from build123d import *

# Parameters (mm, degrees)
SKETCH1_R           = 2
SKETCH1_R_2         = 5
SKETCH1_R_3         = 1.55
SKETCH1_W           = 20
SKETCH1_H           = 7
BOSS_EXTRUDE1_DEPTH = 6


with BuildPart() as part:
    # Sketch1 → Boss-Extrude1 (new body)
    with BuildSketch(Plane.XY):
        with BuildLine():
            Line((95, -44.105037838), (35, -44.105037838))
            ThreePointArc((35, -44.105037838), (27.928932188, -41.17610565), (25, -34.105037838))
            Line((25, -34.105037838), (25, 41.105037842))
            ThreePointArc((25, 41.105037842), (25.732233047, 42.872804795), (27.5, 43.605037842))
            Line((27.5, 43.605037842), (45.75, 43.605037842))
            ThreePointArc((45.75, 43.605037842), (47.517766953, 44.337270889), (48.25, 46.105037842))
            Line((48.25, 46.105037842), (48.25, 61.605037842))
            ThreePointArc((48.25, 61.605037842), (47.517766953, 63.372804795), (45.75, 64.105037842))
            Line((45.75, 64.105037842), (-45.75, 64.105037842))
            ThreePointArc((-45.75, 64.105037842), (-47.517766953, 63.372804795), (-48.25, 61.605037842))
            Line((-48.25, 61.605037842), (-48.25, 46.105037842))
            ThreePointArc((-48.25, 46.105037842), (-47.517766953, 44.337270889), (-45.75, 43.605037842))
            Line((-45.75, 43.605037842), (-27.5, 43.605037842))
            ThreePointArc((-27.5, 43.605037842), (-25.732233047, 42.872804795), (-25, 41.105037842))
            Line((-25, 41.105037842), (-25, -34.105037838))
            ThreePointArc((-25, -34.105037838), (-27.928932188, -41.17610565), (-35, -44.105037838))
            Line((-35, -44.105037838), (-95, -44.105037838))
            ThreePointArc((-95, -44.105037838), (-102.071067812, -47.033970026), (-105, -54.105037838))
            Line((-105, -54.105037838), (-105, -65.855037838))
            Line((-105, -65.855037838), (-103.4, -65.855037838))
            Line((-103.4, -65.855037838), (-103.4, -92.355037838))
            Line((-103.4, -92.355037838), (-105, -92.355037838))
            Line((-105, -92.355037838), (-105, -104.105037838))
            ThreePointArc((-105, -104.105037838), (-102.071067812, -111.17610565), (-95, -114.105037838))
            Line((-95, -114.105037838), (95, -114.105037838))
            ThreePointArc((95, -114.105037838), (102.071067812, -111.17610565), (105, -104.105037838))
            Line((105, -104.105037838), (105, -92.355037838))
            Line((105, -92.355037838), (103.4, -92.355037838))
            Line((103.4, -92.355037838), (103.4, -65.855037838))
            Line((103.4, -65.855037838), (105, -65.855037838))
            Line((105, -65.855037838), (105, -54.105037838))
            ThreePointArc((105, -54.105037838), (102.071067812, -47.033970026), (95, -44.105037838))
        make_face()
        with Locations((80.75, -87.105037838)):
            Circle(SKETCH1_R, mode=Mode.SUBTRACT)
        with Locations((87.75, -79.105037838)):
            Circle(SKETCH1_R_2, mode=Mode.SUBTRACT)
        with Locations((94.75, -71.105037838)):
            Circle(SKETCH1_R, mode=Mode.SUBTRACT)
        with Locations((80.75, -71.105037838)):
            Circle(SKETCH1_R, mode=Mode.SUBTRACT)
        with Locations((-80.75, -71.105037838)):
            Circle(SKETCH1_R, mode=Mode.SUBTRACT)
        with Locations((-94.75, -71.105037838)):
            Circle(SKETCH1_R, mode=Mode.SUBTRACT)
        with Locations((-87.75, -79.105037838)):
            Circle(SKETCH1_R_2, mode=Mode.SUBTRACT)
        with Locations((-80.75, -87.105037838)):
            Circle(SKETCH1_R, mode=Mode.SUBTRACT)
        with Locations((-18.894331083, -54.378109012)):
            Circle(SKETCH1_R_3, mode=Mode.SUBTRACT)
        with Locations((18.605668917, -16.878109012)):
            Circle(SKETCH1_R_3, mode=Mode.SUBTRACT)
        with Locations((-18.894331083, -16.878109012)):
            Circle(SKETCH1_R_3, mode=Mode.SUBTRACT)
        with Locations((18.605668917, -54.378109012)):
            Circle(SKETCH1_R_3, mode=Mode.SUBTRACT)
        with Locations((19.746744501, 21.488147141)):
            Circle(SKETCH1_R, mode=Mode.SUBTRACT)
        with Locations((-19.253255499, 21.488147141)):
            Circle(SKETCH1_R, mode=Mode.SUBTRACT)
        with Locations((-94.75, -87.105037838)):
            Circle(SKETCH1_R, mode=Mode.SUBTRACT)
        with Locations((94.75, -87.105037838)):
            Circle(SKETCH1_R, mode=Mode.SUBTRACT)
        with BuildLine():
            Line((-41.45, 49.205037842), (-24.55, 49.205037842))
            ThreePointArc((-24.55, 49.205037842), (-22.75, 47.405037842), (-24.55, 45.605037842))
            Line((-24.55, 45.605037842), (-41.45, 45.605037842))
            ThreePointArc((-41.45, 45.605037842), (-43.25, 47.405037842), (-41.45, 49.205037842))
        make_face(mode=Mode.SUBTRACT)
        with BuildLine():
            Line((41.45, 45.605037842), (24.55, 45.605037842))
            ThreePointArc((24.55, 45.605037842), (22.75, 47.405037842), (24.55, 49.205037842))
            Line((24.55, 49.205037842), (41.45, 49.205037842))
            ThreePointArc((41.45, 49.205037842), (43.25, 47.405037842), (41.45, 45.605037842))
        make_face(mode=Mode.SUBTRACT)
        with Locations((0, 43.605037842)):
            Rectangle(SKETCH1_W, SKETCH1_H, mode=Mode.SUBTRACT)
    extrude(amount=BOSS_EXTRUDE1_DEPTH)


solid = part.part
For this review, take the finished solid that the model builds, in its own axes (mm). A direction names the side the tool comes from. Give positions to 0.01 mm unless a question says otherwise; leave off trailing zeros. Order: outer loops, then holes, each group sorted by start corner. A loop starts at its lowest first (then second) coordinate and runs counter-clockwise, first axis right, second up. Notation, with made-up numbers: (-20.75, 15) -> (-10.75, 15) arc R26 cw to (-10.75, 52) -> close; hole circle Ø3 at (40, 2.5). An arc over 180 degrees is marked (long way). Write item = value, one per line.
1) We need section D-D, the plane z = 5.05. Count the separate pieces of the cut face and the enclosed holes in it, and give its area (3 significant figures).
Findings:
separate_pieces = 1
enclosed_holes = 19
area = 20,300 mm^2
2) We need section C-C, the plane x = -87.75. Give the boundary of the cut face in (y, z).
Findings:
outline = (-114.11, 0) -> (-84.11, 0) -> (-84.11, 6) -> (-114.11, 6) -> close; (-74.11, 0) -> (-44.11, 0) -> (-44.11, 6) -> (-74.11, 6) -> close
3) We need section B-B, the plane y = -81.5. Give the boundary of the cut face in (x, z).
Findings:
outline = (-103.4, 0) -> (-92.14, 0) -> (-92.14, 6) -> (-103.4, 6) -> close; (-83.36, 0) -> (83.36, 0) -> (83.36, 6) -> (-83.36, 6) -> close; (92.14, 0) -> (103.4, 0) -> (103.4, 6) -> (92.14, 6) -> close
4) For faces 1 (the face through (-48.25, 54, 3)), 2 (the face through (28.007, -41.253, 2.958)), 3 (the face through (10, 44, 3)), 4 (the face through (-25, 4, 3)), list the 3-axis set-ups (+Z, -Z, +X, -X, +Y, -Y) from which the entire face can be reached by the end or side of a thin tool; tool diameter is ignored.
Findings:
face_1 = +Z, -Z, -X, +Y
face_2 = +Z, -Z, +X
face_3 = +Z, -Z
face_4 = +Z, -Z, -X
5) Insertion check: pin 1 (4.5 mm diameter, centred on x = -94.75, y = -71.11, fed in from +Z); pin 2 (2 mm diameter, centred on y = 14, z = 1, fed in from -X); pin 3 (3 mm diameter, centred on y = 12, z = 3.5, fed in from +X); pin 4 (1.3 mm diameter, centred on x = -104, z = 2.5, fed in from +Y). Each pin has a flat end and moves straight along its axis. Give the tip position at first contact, or say it passes through.
Findings:
pin_1 = 6
pin_2 = -25
pin_3 = 25
pin_4 = -48.6
6) Draft analysis for pull direction X (two halves, no side actions). For faces 5 (the face through (36, 43.605, 3)), 6 (the face through (0, 47.105, 3)), 7 (the face through (-103.4, -79, 3)), state which applies: pulls with the +X half, pulls with the -X half, needs draft (parallel to the pull), parting line crosses it, or undercut.
Findings:
face_5 = needs draft
face_6 = undercut
face_7 = pulls with the -X half
7) To check wall thickness, follow L1, parallel to Y at x = -81, z = 4.4; L2, parallel to X at y = -79.5, z = 1.55; L3, parallel to X at y = 20, z = 5.3. State the ranges of each line that lie inside material, in increasing order. Write a range as from..to.
Findings:
L1 = -114.11..-89.09, -85.12..-73.09, -69.12..-44.11
L2 = -103.4..-92.73, -82.77..82.77, 92.73..103.4
L3 = -25..-20.59, -17.92..18.41, 21.08..25
8) We need section A-A, the plane x = 6. Give the boundary of the cut face in (y, z), and give its area (3 significant figures).
Findings:
outline = (-114.11, 0) -> (40.11, 0) -> (40.11, 6) -> (-114.11, 6) -> close; (47.11, 0) -> (64.11, 0) -> (64.11, 6) -> (47.11, 6) -> close
area = 1,030 mm^2
